Here's how the part is built. I have some questions about the finished solid (model axes, mm). A direction names the side the tool comes from. Give positions to 0.01 mm unless a question says otherwise; leave off trailing zeros. Write each loop counter-clockwise with the first axis right and the second up, starting at its lowest first coordinate (ties: lowest second). Pieces come first, ordered by that corner, then holes. Notation, with made-up numbers: (-8, 78.5) -> (-2, 78.5) arc R24 cw to (-2, 89.5) -> close; hole circle Ø11 at (28, 31.25). An arc over 180 degrees is marked (long way). Use one line per item in the form item = value.
```python
from build123d import *

# Parameters (mm, degrees)
SKETCH2_R           = 23
BOSS_EXTRUDE1_DEPTH = 10
BOSS_EXTRUDE2_DEPTH = 80
SKETCH5_R           = 0.5
BOSS_EXTRUDE3_DEPTH = 5


with BuildPart() as part:
    # Sketch2 → Boss-Extrude1 (new body)
    with BuildSketch(Plane.XY):
        Circle(SKETCH2_R)
        Polygon((-6.3, 0), (-3.15, -5.455960044), (3.15, -5.455960044), (6.3, 0), (3.15, 5.455960044), (-3.15, 5.455960044), align=None, mode=Mode.SUBTRACT)
    extrude(amount=BOSS_EXTRUDE1_DEPTH)

    # Sketch2_2 → Boss-Extrude2 (add)
    with BuildSketch(Plane.XY):
        Polygon((3.15, 5.455960044), (-3.15, 5.455960044), (-6.3, 0), (-3.15, -5.455960044), (3.15, -5.455960044), (6.3, 0), align=None)
    extrude(amount=BOSS_EXTRUDE2_DEPTH)

    # Sketch5 → Boss-Extrude3 (add)
    with BuildSketch(Plane(origin=(0, 0, 0), x_dir=(-1, 0, 0), z_dir=(0, 0, -1))):
        with Locations(Location((-7.068259509, 7.073875, 0), (0, 0, 180))):
            Circle(SKETCH5_R)
        with Locations(Location((0, 10, 0), (0, 0, 180))):
            Circle(SKETCH5_R)
        with Locations(Location((7.068259509, 7.073875, 0), (0, 0, 180))):
            Circle(SKETCH5_R)
        with Locations(Location((-7.07948603, -7.06263956, 0), (0, 0, 180))):
            Circle(SKETCH5_R)
        with Locations(Location((-9.999996847, 0.007941503, 0), (0, 0, 180))):
            Circle(SKETCH5_R)
        with Locations(Location((-0.015888246, -10, 0), (0, 0, 180))):
            Circle(SKETCH5_R)
        with Locations(Location((7.057007753, -7.08509997, 0), (0, 0, 180))):
            Circle(SKETCH5_R)
        with Locations(Location((9.961481677, -0.007916121, 0), (0, 0, 180))):
            Circle(SKETCH5_R)
    extrude(amount=BOSS_EXTRUDE3_DEPTH)


solid = part.part
```
Q1. I want a section at A-A, the plane z = 38. Write out the boundary of the cut face in (x, y), and give its area (3 significant figures).
Result set:
outline = (-6.3, 0) -> (-3.15, -5.46) -> (3.15, -5.46) -> (6.3, 0) -> (3.15, 5.46) -> (-3.15, 5.46) -> close
area = 103 mm2
Q2. I want a section at C-C, the plane x = -8.5. Write out the boundary of the cut face in (y, z).
Result set:
outline = (-21.37, 0) -> (21.37, 0) -> (21.37, 10) -> (-21.37, 10) -> close
Q3. If I drill on line 1 along Z through (x, y) = (-9.5, 20.5); line 2 along Z through (x, y) = (3, -3); line 3 along Y through (x, z) = (-4, 27), over which ranges is the centre line in solid material (lowest first)? Write a range as from..to.
Result set:
line_1 = 0..10
line_2 = 0..80
line_3 = -3.98..3.98
Q4. Which directions (+Z, -Z, +X, -X, +Y, -Y) give clear straight access to the entire face, cutting with the end or side of a thin tool? Please do faces 1 (the face through (5, -5, 10)), 2 (the face through (0, 5.456, 45)), 3 (the face through (0, 0, 0)).
Result set:
face_1 = +Z
face_2 = +Z, +X, -X, +Y
face_3 = -Z
Q5. I want a section at B-B, the plane y = 4.5. Write out the boundary of the cut face in (x, z).
Result set:
outline = (-22.56, 0) -> (22.56, 0) -> (22.56, 10) -> (3.7, 10) -> (3.7, 80) -> (-3.7, 80) -> (-3.7, 10) -> (-22.56, 10) -> close
Q6. Will these pins go through, and if not, where does the flat tip stop? pin 1 Ø3 at (x, z) = (1, 55.5) entering from -Y; pin 2 Ø7 at (x, z) = (-1.5, 57) entering from +Y; pin 3 Ø6 at (y, z) = (-10, 35) entering from +X; pin 4 Ø1.5 at (x, y) = (-17, -14) entering from -Z.
Result set:
pin_1 = -5.46
pin_2 = 5.46
pin_3 = through
pin_4 = 0
Q7. I want a section at D-D, the plane z = 3.5. Write out the boundary of the cut face in (x, y), and give its area (3 significant figures).
Result set:
outline = circle Ø46 at (0, 0)
area = 1,660 mm2
